from build123d import *

# Parameters (mm, degrees)
SKETCH3_W                       = 55.92
SKETCH3_H                       = 48.2
BOSS_EXTRUDE1_DEPTH             = 8
BOSS_EXTRUDE2_DEPTH             = 95
SKETCH5_R                       = 2.75
SKETCH5_W                       = 40.7
SKETCH5_H                       = 64.8
CUT_EXTRUDE1_DEPTH              = 124.599095466
BOSS_EXTRUDE4_DEPTH             = 55.92
SKETCH9_R                       = 42.5
CUT_EXTRUDE2_DEPTH              = 229.287727222
SKETCH10_W                      = 18
SKETCH10_H                      = 140
SKETCH10_W_2                    = 13.92
SKETCH10_H_2                    = 100
CUT_EXTRUDE3_DEPTH              = 216.852487593
SKETCH11_W                      = 48.42
SKETCH11_H                      = 10.7
BOSS_EXTRUDE5_DEPTH             = 16
SKETCH12_R                      = 0.875
CUT_EXTRUDE7_DEPTH              = 8
CUT_EXTRUDE8_START              = -43.2
SKETCH12_3_R                    = 0.875
CUT_EXTRUDE8_DEPTH              = 5
FILLET3_R                       = 1
CUT_EXTRUDE9_REACH              = 218.008
SKETCH14_R                      = 1.6
SKETCH15_W                      = 11
SKETCH15_H                      = 15
BOSS_EXTRUDE6_DEPTH             = 20
BOSS_EXTRUDE6_DIRECTION_2_REACH = 217.827
CUT_EXTRUDE10_REACH             = 230.242
SKETCH16_R                      = 1.6
CUT_EXTRUDE13_DEPTH             = 216.826567209
CUT_EXTRUDE13_DEPTH_BACK        = 216.826567209
SKETCH17_W                      = 258.17245833
SKETCH17_H                      = 778.313168381
CUT_EXTRUDE14_DEPTH             = 15


with BuildPart() as part:
    # Sketch3 → Boss-Extrude1 (new body)
    with BuildSketch(Plane(origin=(0, 0, 0), x_dir=(1, 0, 0), z_dir=(0, 1, 0))):
        with Locations((-27.96, 24.1)):
            Rectangle(SKETCH3_W, SKETCH3_H)
    extrude(amount=BOSS_EXTRUDE1_DEPTH)

    # Sketch4 → Boss-Extrude2 (add)
    with BuildSketch(Plane(origin=(0, 8, 0), x_dir=(1, 0, 0), z_dir=(0, 1, 0))):
        Polygon((-55.92, 0), (-55.92, 48.2), (0, 48.2), (0, 40.7), (-48.42, 40.7), (-48.42, 0), align=None)
    extrude(amount=BOSS_EXTRUDE2_DEPTH)

    # Sketch5 → Cut-Extrude1 (cut, through all)
    with BuildSketch(Plane(origin=(-48.42, 0, 0), x_dir=(0, 0, -1), z_dir=(1, 0, 0))):
        with Locations((17.2, 12.5)):
            Circle(SKETCH5_R)
        with Locations((34.2, 12.5)):
            Circle(SKETCH5_R)
        with Locations(Location((34.2, 87.5, 0), (0, 0, 180))):
            Circle(SKETCH5_R)
        with Locations(Location((17.2, 87.5, 0), (0, 0, 180))):
            Circle(SKETCH5_R)
        with Locations((20.35, 50)):
            Rectangle(SKETCH5_W, SKETCH5_H)
    extrude(amount=-CUT_EXTRUDE1_DEPTH, mode=Mode.SUBTRACT)

    # Sketch8 → Boss-Extrude4 (add)
    with BuildSketch(Plane(origin=(0, 0, 0), x_dir=(0, 0, -1), z_dir=(1, 0, 0))):
        Polygon((40.7, 103), (40.7, 203), (45.7, 203), (88.2, 153), (48.2, 24), (48.2, 103), align=None)
    extrude(amount=-BOSS_EXTRUDE4_DEPTH)

    # Sketch9 → Cut-Extrude2 (cut, through all)
    with BuildSketch(Plane(origin=(0, 0, 0), x_dir=(0, 0, -1), z_dir=(1, 0, 0))):
        with Locations((22.577976258, 153)):
            Circle(SKETCH9_R)
    extrude(amount=-CUT_EXTRUDE2_DEPTH, mode=Mode.SUBTRACT)

    # Sketch10 → Cut-Extrude3 (cut, through all)
    with BuildSketch(Plane.XY.offset(-40.7)):
        with Locations((-21, 133)):
            Rectangle(SKETCH10_W, SKETCH10_H)
        with Locations((-48.96, 153)):
            Rectangle(SKETCH10_W_2, SKETCH10_H_2)
    extrude(amount=-CUT_EXTRUDE3_DEPTH, mode=Mode.SUBTRACT)

    # Sketch11 → Boss-Extrude5 (add)
    with BuildSketch(Plane(origin=(0, 8, 0), x_dir=(1, 0, 0), z_dir=(0, 1, 0))):
        with Locations((-24.21, 5.35)):
            Rectangle(SKETCH11_W, SKETCH11_H)
    extrude(amount=BOSS_EXTRUDE5_DEPTH)

    # Sketch12 → Cut-Extrude7 (cut)
    with BuildSketch(Plane.XY):
        with Locations((-39.96, 8.15)):
            Circle(SKETCH12_R)
        with Locations((-39.96, 20.15)):
            Circle(SKETCH12_R)
        with Locations((-27.96, 8.15)):
            Circle(SKETCH12_R)
        with Locations(Location((-15.96, 8.15, 0), (0, 0, 180))):
            Circle(SKETCH12_R)
        with Locations(Location((-15.96, 20.15, 0), (0, 0, 180))):
            Circle(SKETCH12_R)
    extrude(amount=-CUT_EXTRUDE7_DEPTH, mode=Mode.SUBTRACT)

    # Sketch12<3> → Cut-Extrude8 (cut)
    with BuildSketch(Plane.XY.offset(CUT_EXTRUDE8_START)):
        with Locations((-39.96, 8.15)):
            Circle(SKETCH12_3_R)
        with Locations((-39.96, 20.15)):
            Circle(SKETCH12_3_R)
        with Locations((-27.96, 8.15)):
            Circle(SKETCH12_3_R)
        with Locations(Location((-15.96, 8.15, 0), (0, 0, 180))):
            Circle(SKETCH12_3_R)
        with Locations(Location((-15.96, 20.15, 0), (0, 0, 180))):
            Circle(SKETCH12_3_R)
    extrude(amount=-CUT_EXTRUDE8_DEPTH, mode=Mode.SUBTRACT)

    # Fillet3
    fillet3_edges = [part.edges().sort_by_distance(p)[0] for p in [
        (-36, 191.442713945, -40.7),
        (-6, 191.442713945, -40.7),
        (-42, 153, -65.077976258),
        (-12, 153, -65.077976258),
        (-30, 153, -65.077976258),
        (-36, 153, -88.2),
        (-6, 153, -88.2),
        (-48.96, 103, -72.696124031),
        (-21, 63, -60.293023256),
        (-36, 203, -45.7),
        (-6, 203, -45.7),
        (-36, 203, -40.7),
        (-6, 203, -40.7),
        (-30, 178, -66.95),
        (-30, 108, -74.246511628),
        (-30, 63, -50.496511628),
        (-12, 178, -66.95),
        (-12, 108, -74.246511628),
        (-12, 203, -43.2),
        (-12, 88.778643027, -40.7),
        (-30, 88.778643027, -40.7),
        (-21, 63, -40.7),
        (-30, 197.221356973, -40.7),
        (-12, 197.221356973, -40.7),
        (-30, 203, -43.2),
        (-12, 63, -50.496511628),
        (-42, 178, -66.95),
        (-42, 128, -80.448062016),
        (-42, 203, -43.2),
        (-42, 197.221356973, -40.7),
        (-45.21, 103, -40.7),
        (-42, 108.778643027, -40.7),
        (-42, 103, -56.698062016),
        (-48.42, 17.6, -25.7),
        (-48.42, 8, -25.7),
        (0, 8, -25.7),
        (-48.42, 20.8, -10.7),
        (-24.21, 8, -10.7),
        (-48.42, 92.7, 0),
        (0, 16, -10.7),
        (-48.42, 12.8, -10.7),
        (-48.42, 20.8, 0),
        (-24.21, 8, -40.7),
        (0, 24, -5.35),
        (-24.21, 24, -10.7),
        (-48.42, 24, -5.35),
        (-24.21, 24, 0),
        (-48.42, 92.7, -40.7),
        (0, 197.221356973, -40.7),
        (-52.17, 103, 0),
        (-48.42, 103, -20.35),
        (-48.42, 12.8, -40.7),
        (-55.92, 8.8, 0),
        (-27.96, 0, -48.2),
        (-52.17, 17.6, 0),
        (-55.92, 82.4, -20.35),
        (-52.17, 82.4, 0),
        (-55.92, 50, -40.7),
        (-52.17, 82.4, -40.7),
        (-55.92, 17.6, -20.35),
        (-52.17, 17.6, -40.7),
        (-48.42, 17.6, -5.35),
        (0, 0, -24.1),
        (-48.42, 82.4, -20.35),
        (-27.96, 0, 0),
        (-55.92, 0, -24.1),
        (-55.92, 103, -36.348062016),
        (-55.92, 12, -48.2),
        (0, 12, -48.2),
        (-55.92, 63.5, -60.448062016),
        (-27.96, 24, -48.2),
        (0, 88.5, -68.2),
        (0, 178, -66.95),
        (0, 203, -43.2),
        (0, 12, 0),
        (-55.92, 92.7, 0),
        (0, 61.278643027, -40.7),
        (-6, 114.557286055, -40.7),
        (0, 153, -65.077976258),
        (-36, 114.557286055, -40.7),
    ]]
    fillet(fillet3_edges, radius=FILLET3_R)

    # Cut-Extrude9: up to this face of the body (flat: up to its plane)
    cut_extrude9_end = Plane(part.part.faces().sort_by_distance((-26.9866887, 11.661518577, 0))[0])
    # Sketch14 → Cut-Extrude9 (cut, up to the picked face)
    with BuildSketch(Plane(origin=(0, 0, -48.2), x_dir=(-1, 0, 0), z_dir=(0, 0, -1)), mode=Mode.PRIVATE) as cut_extrude9_sk1:
        with Locations((4, 17.228518844)):
            Circle(SKETCH14_R)
    cut_extrude9_tool1 = split(extrude(cut_extrude9_sk1.sketch, amount=-CUT_EXTRUDE9_REACH, mode=Mode.PRIVATE), bisect_by=cut_extrude9_end, keep=Keep.BOTH, mode=Mode.PRIVATE)
    add(cut_extrude9_tool1.solids().sort_by(Axis((-4, 17.228519, -48.2), (0, 0, 1)))[0], mode=Mode.SUBTRACT)

    # Sketch15 → Boss-Extrude6 (add)
    with BuildSketch(Plane.XY.offset(-40.7)):
        with Locations((-5.5, 73)):
            Rectangle(SKETCH15_W, SKETCH15_H)
    extrude(amount=BOSS_EXTRUDE6_DEPTH)

    # Sketch15 → Boss-Extrude6 direction 2 (add, up to next)
    with BuildSketch(Plane.XY.offset(-40.7), mode=Mode.PRIVATE) as boss_extrude6_direction_2_sk1:
        with Locations((-5.5, 73)):
            Rectangle(SKETCH15_W, SKETCH15_H)
    boss_extrude6_direction_2_tool1 = extrude(boss_extrude6_direction_2_sk1.sketch, amount=-BOSS_EXTRUDE6_DIRECTION_2_REACH, mode=Mode.PRIVATE) - part.part
    add(boss_extrude6_direction_2_tool1.solids().sort_by_distance((-5.5, 73, -40.7))[0])

    # Sketch16 → Cut-Extrude10 (cut, up to next)
    with BuildSketch(Plane(origin=(0, 0, 0), x_dir=(0, 0, -1), z_dir=(1, 0, 0)), mode=Mode.PRIVATE) as cut_extrude10_sk1:
        with Locations((25.69, 74.3258878)):
            Circle(SKETCH16_R)
    cut_extrude10_tool1 = extrude(cut_extrude10_sk1.sketch, amount=-CUT_EXTRUDE10_REACH, mode=Mode.PRIVATE) & part.part
    # Sketch16 → Cut-Extrude10 (cut, up to next)
    with BuildSketch(Plane(origin=(0, 0, 0), x_dir=(0, 0, -1), z_dir=(1, 0, 0)), mode=Mode.PRIVATE) as cut_extrude10_sk2:
        with Locations((50.69, 74.3258878)):
            Circle(SKETCH16_R)
    cut_extrude10_tool2 = extrude(cut_extrude10_sk2.sketch, amount=-CUT_EXTRUDE10_REACH, mode=Mode.PRIVATE) & part.part
    add(cut_extrude10_tool1.solids().sort_by_distance((0, 74.325888, -25.69))[0], mode=Mode.SUBTRACT)
    add(cut_extrude10_tool2.solids().sort_by_distance((0, 74.325888, -50.69))[0], mode=Mode.SUBTRACT)

    # Sketch17 → Cut-Extrude13 (cut, two sides: drawn at the far end of the back side and taken through both)
    with BuildSketch(Plane.XY.offset(-40.7).offset(-CUT_EXTRUDE13_DEPTH_BACK)):
        with Locations((-159.086229165, 140.248603605)):
            Rectangle(SKETCH17_W, SKETCH17_H)
    extrude(amount=CUT_EXTRUDE13_DEPTH + CUT_EXTRUDE13_DEPTH_BACK, mode=Mode.SUBTRACT)

    # Sketch21 → Cut-Extrude14 (cut)
    with BuildSketch(Plane(origin=(-30, 0, 0), x_dir=(0, 0, -1), z_dir=(1, 0, 0))):
        Polygon((45.7, 50), (48.2, 54.330127019), (50.7, 50), align=None)
        Polygon((43.2, 35), (48.2, 35), (45.7, 30.669872981), align=None)
        Polygon((45.7, 2.5), (40.7, 2.5), (43.2, 6.830127019), align=None)
        Polygon((2.85, 20.5), (7.85, 20.5), (5.35, 16.169872981), align=None)
        Polygon((10, 2.5), (5, 2.5), (7.5, 6.830127019), align=None)
    extrude(amount=CUT_EXTRUDE14_DEPTH, mode=Mode.SUBTRACT)


solid = part.part
Read the model definition and answer for the solid it produces. Units are mm, in the model's axes. A direction names the side the tool comes from. Round coordinates to 2 decimals unless told otherwise and drop trailing zeros.
1) Straight lines are drawn through the part: L1, parallel to Y at x = -28, z = -3.5; L2, parallel to Y at x = -17, z = -47; L3, parallel to Y at x = -14, z = -26. For each, find the intervals that lie inside material, in ascending order.
2) The part is cut by section A-A on x = -19.5. Give the number of separate pieces and of enclosed holes in the cut face, plus the area to 3 significant figures.
3) The mould has two halves that part along Y. Classify faces 5 (the face through (-16, 0, -24)), 6 (the face through (-6, 197, -40.7)), 7 (the face through (-15, 19, -5)): released by +Y, released by -Y, zero draft, split by the parting line, or undercut.
4) For faces 1 (the face through (-11, 73, -31)), 2 (the face through (-6, 97, -40.7)), 3 (the face through (-12, 117, -59)), 4 (the face through (-21, 63, -50)), determine the directions among +Z, -Z, +X, -X, +Y, -Y from which every point of the face is accessible in a straight line to the end or side of a thin tool.
5) Flat-ended cylindrical pins translate along their axes: pin 1 (8 mm diameter, centred on y = 62.5, z = -35.5, fed in from -X); pin 2 (4.5 mm diameter, centred on x = -15.5, z = -3.5, fed in from +Y); pin 3 (1.3 mm diameter, centred on y = 18.5, z = -5.5, fed in from -X); pin 4 (4 mm diameter, centred on x = -21, z = -63, fed in from -Y). Find the tip coordinate at first contact, or state that the pin passes through.
Resolved:
1. L1: y = 0 to 7.28, 9.02 to 19.37, 20.5 to 24
1. L2: y = 0 to 32.92, 35 to 50, 52.25 to 63
1. L3: y = 0 to 8
2. separate pieces: 1
2. enclosed holes: 5
2. area: 1,150 mm2
3. face 5: released by -Y
3. face 6: zero draft
3. face 7: undercut
4. face 1: +Z, -X, +Y
4. face 2: +Z, +X, -X, +Y
4. face 3: +Z, -Z, -X, +Y
4. face 4: +Z, -Z, +Y
5. pin 1: stops at x = -11
5. pin 2: stops at y = 24
5. pin 3: stops at x = -15
5. pin 4: passes through
